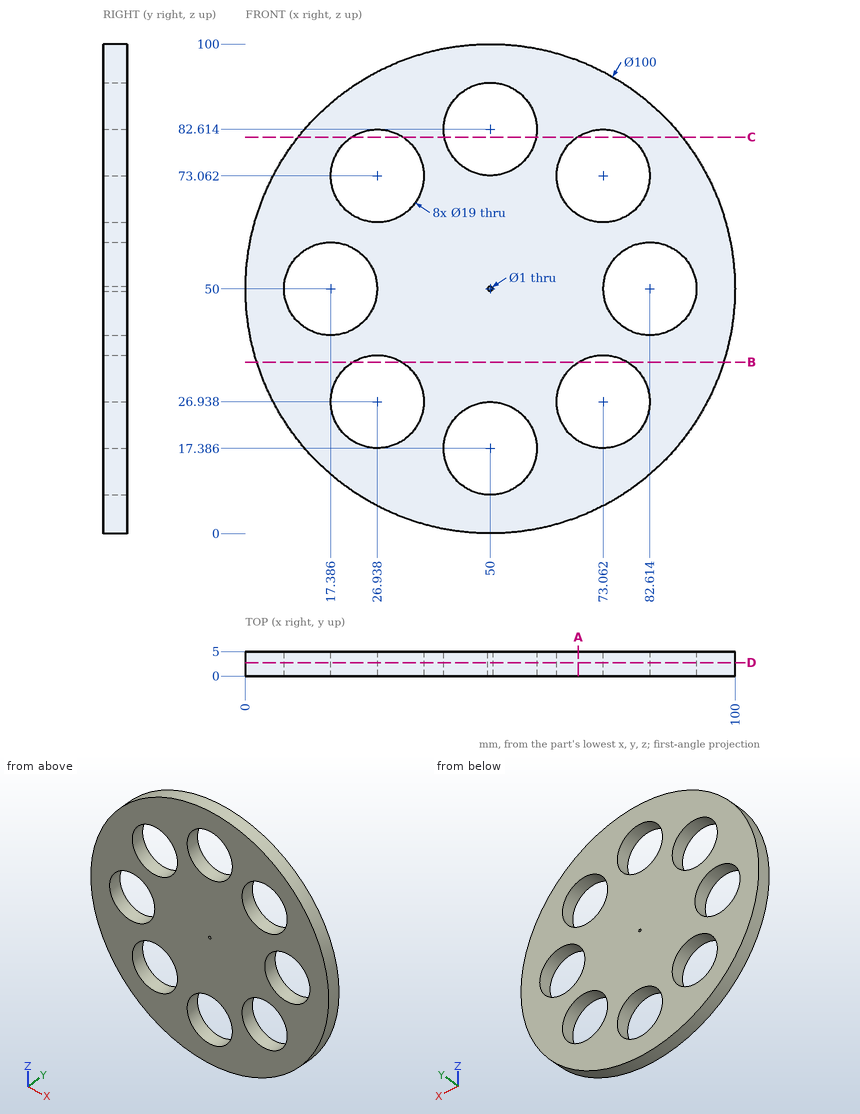
Here's the drawing with two shaded views (mm, measured from the low corner). I have some questions. Give positions to 0.01 mm unless a question says otherwise; leave off trailing zeros. Order: outer loops, then holes, each group sorted by start corner. A loop starts at its lowest first (then second) coordinate and runs counter-clockwise, first axis right, second up.
Q1. Suppose I cut it at B-B, the plane z = 35. Write out the boundary of the cut face in (x, y).
Q2. Suppose I cut it at D-D, the plane y = 2.75. Count the separate pieces of the cut face and the enclosed holes in it.
Q3. Suppose I cut it at C-C, the plane z = 81. Write out the boundary of the cut face in (x, y).
Q4. If I drill on line 1 along X through (y, z) = (1, 50); line 2 along X through (y, z) = (1.35, 51), over which ranges is the centre line in solid material (lowest first)?
Q5. I'm going to push flat-ended pins straight in: P1, Ø1, axis at y = 1, z = 84, coming from the +X side; P2, Ø1, axis at y = 3, z = 33.5, coming from the +X side; P3, Ø1, axis at y = 4, z = 59.5, coming from the +X side; P4, Ø11.5, axis at x = 50, z = 82.61, coming from the +Y side. Where does each tip first touch, or does it pass through?
Q6. Suppose I cut it at A-A, the plane x = 68. Write out the boundary of the cut face in (y, z).
Solution:
1. outline: (2.3, 0) - (21.91, 0) - (21.91, 5) - (2.3, 5) - close; (31.96, 0) - (68.04, 0) - (68.04, 5) - (31.96, 5) - close; (78.09, 0) - (97.7, 0) - (97.7, 5) - (78.09, 5) - close
2. separate pieces: 1
2. enclosed holes: 9
3. outline: (10.77, 0) - (21.72, 0) - (21.72, 5) - (10.77, 5) - close; (32.16, 0) - (40.64, 0) - (40.64, 5) - (32.16, 5) - close; (59.36, 0) - (67.84, 0) - (67.84, 5) - (59.36, 5) - close; (78.28, 0) - (89.23, 0) - (89.23, 5) - (78.28, 5) - close
4. line 1: x = 0 to 7.89, 26.89 to 49.5, 50.5 to 73.11, 92.11 to 100
4. line 2: x = 0.01 to 7.94, 26.83 to 73.17, 92.06 to 99.99
5. P1: stops at x = 87.12
5. P2: stops at x = 97.37
5. P3: stops at x = 99.18
5. P4: passes through
6. outline: (0, 3.35) - (5, 3.35) - (5, 18.9) - (0, 18.9) - close; (0, 34.98) - (5, 34.98) - (5, 65.02) - (0, 65.02) - close; (0, 81.1) - (5, 81.1) - (5, 96.65) - (0, 96.65) - close
